```python
from build123d import *

# Parameters (mm, degrees)
BOSS_EXTRUDE1_DEPTH = 6


with BuildPart() as part:
    # Sketch1 → Boss-Extrude1 (new body)
    with BuildSketch(Plane.XY):
        Polygon((349.805861239, 49.832080259), (349.805861239, 56.546676312), (337.582956824, 56.546676312), (337.582956824, 94.832680829), (342.594184557, 99.843908562), (359.928534592, 99.843908562), (364.939762315, 94.832680839), (364.939762315, 73.014449736), (403.254521851, 61.257454897), (403.254521851, 56.546676274), (392.232066466, 56.546676274), (392.232066466, 49.832080221), (403.26125874, 49.832080221), (403.26125874, 24.580912459), (394.140824266, 24.580912459), (337.582956824, 45.121301639), (337.582956824, 49.832080259), align=None)
        Polygon((396.07235895, 38.585081223), (396.445988279, 38.87177709), (396.881088847, 39.052001647), (397.348009271, 39.113472887), (397.814929694, 39.052001647), (398.250030262, 38.87177709), (398.623659591, 38.585081223), (398.910355458, 38.211451895), (399.090580014, 37.776351326), (399.152051254, 37.309430903), (399.090580014, 36.842510479), (398.910355458, 36.407409911), (398.623659591, 36.033780583), (398.250030262, 35.747084715), (397.814929694, 35.566860159), (397.348009271, 35.505388919), (396.881088847, 35.566860159), (396.445988279, 35.747084715), (396.07235895, 36.033780583), (395.785663083, 36.407409911), (395.605438527, 36.842510479), (395.543967287, 37.309430903), (395.605438527, 37.776351326), (395.785663083, 38.211451895), align=None, mode=Mode.SUBTRACT)
        Polygon((351.375405933, 69.514088989), (351.436877173, 69.047168565), (351.617101729, 68.612067997), (351.903797596, 68.238438669), (352.277426924, 67.951742801), (352.712527493, 67.771518245), (353.179447916, 67.710047005), (353.64636834, 67.771518245), (354.081468908, 67.951742801), (354.455098237, 68.238438669), (354.741794104, 68.612067997), (354.92201866, 69.047168565), (354.9834899, 69.514088989), (354.92201866, 69.981009412), (354.741794104, 70.416109981), (354.455098237, 70.789739309), (354.081468908, 71.076435176), (353.64636834, 71.256659733), (353.179447916, 71.318130973), (352.712527493, 71.256659733), (352.277426924, 71.076435176), (351.903797596, 70.789739309), (351.617101729, 70.416109981), (351.436877173, 69.981009412), align=None, mode=Mode.SUBTRACT)
        Polygon((372.381509854, 54.465028594), (372.007880526, 54.751724461), (371.572779958, 54.931949018), (371.105859534, 54.993420258), (370.638939111, 54.931949018), (370.203838542, 54.751724461), (369.830209214, 54.465028594), (369.543513347, 54.091399266), (369.36328879, 53.656298697), (369.30181755, 53.189378274), (369.36328879, 52.72245785), (369.543513347, 52.287357282), (369.830209214, 51.913727954), (370.203838542, 51.627032087), (370.638939111, 51.44680753), (371.105859534, 51.38533629), (371.572779958, 51.44680753), (372.007880526, 51.627032087), (372.381509854, 51.913727954), (372.668205722, 52.287357282), (372.848430278, 52.72245785), (372.909901518, 53.189378274), (372.848430278, 53.656298697), (372.668205722, 54.091399266), align=None, mode=Mode.SUBTRACT)
        Polygon((350.579160049, 82.777243303), (351.409447446, 82.140141376), (352.376337597, 81.739642362), (353.413938539, 81.603039606), (354.45153948, 81.739642362), (355.418429632, 82.140141376), (356.248717028, 82.777243303), (356.885818955, 83.607530699), (357.286317969, 84.574420851), (357.422920725, 85.612021792), (357.286317969, 86.649622733), (356.885818955, 87.616512885), (356.248717028, 88.446800282), (355.418429632, 89.083902209), (354.45153948, 89.484401223), (353.413938539, 89.621003978), (352.376337597, 89.484401223), (351.409447446, 89.083902209), (350.579160049, 88.446800282), (349.942058122, 87.616512885), (349.541559108, 86.649622733), (349.404956353, 85.612021792), (349.541559108, 84.574420851), (349.942058122, 83.607530699), align=None, mode=Mode.SUBTRACT)
    extrude(amount=BOSS_EXTRUDE1_DEPTH)


solid = part.part
```
Geometry check sheet. Reference: the model listing, model coordinates, mm. A direction names the side the tool comes from. Round coordinates to 2 decimals unless told otherwise and drop trailing zeros. Order: outer loops, then holes, each group sorted by start corner. A loop starts at its lowest first (then second) coordinate and runs counter-clockwise, first axis right, second up. Notation, with made-up numbers: (27.5, 46) -> (55.5, 46) arc R16 ccw to (55.5, 67) -> close; hole circle Ø1 at (24.5, 12.25). An arc over 180 degrees is marked (long way). Return JSON: item names as keys, results as strings. Group by question number.
Q1. Section check B-B, the plane z = 4.25. Count the separate pieces of the cut face and the enclosed holes in it, plus the area to 3 significant figures.
Q2. Section check A-A, the plane x = 345.5. Record the boundary of the cut face in (y, z).
Q3. Release check for a two-part mould opening along Y. For faces 4 (the flat face through (344, 56.547, 3)), 5 (the flat face through (364, 63, 0)), 6 (the flat face through (399, 24.581, 3)) record: released by +Y, released by -Y, zero draft, split by the parting line, or undercut.
Q4. Gauge pin test, flat ends, axial feed: pin 1 (3 mm diameter, centred on x = 346.5, z = 2, fed in from -Y); pin 2 (1 mm diameter, centred on x = 375.5, z = 4, fed in from +Y); pin 3 (1.8 mm diameter, centred on y = 88, z = 2.5, fed in from +X); pin 4 (4 mm diameter, centred on x = 365.5, y = 32.5, fed in from +Z). Record the tip position at first contact, or that the pin passes through.
Q5. Material ranges on probe 1 along Y at (x, z) = (398.5, 1.1); probe 2 along X at (y, z) = (77, 4.4); probe 3 along X at (y, z) = (82, 4.75), recorded low to high. Write a range as from..to.
Q6. Section check C-C, the plane x = 377. Record the boundary of the cut face in (y, z), plus the area to 3 significant figures.
Q7. Tool access check on faces 1 (the flat face through (364.94, 84, 3)), 2 (the flat face through (344, 49.832, 3)), 3 (the flat face through (398, 49.832, 3)). Record the directions out of +Z, -Z, +X, -X, +Y, -Y that give a thin tool (end or side, any length) a straight path to the whole face; none if there is none.
Numbers:
{
 "1": {"separate pieces": "1", "enclosed holes": "4", "area": "2,850 mm^2"},
 "2": {"outline": "(42.25, 0) -> (49.83, 0) -> (49.83, 6) -> (42.25, 6) -> close; (56.55, 0) -> (99.84, 0) -> (99.84, 6) -> (56.55, 6) -> close"},
 "3": {"face 4": "undercut", "face 5": "zero draft", "face 6": "released by -Y"},
 "4": {"pin 1": "y = 41.34", "pin 2": "y = 69.93", "pin 3": "x = 364.94", "pin 4": "through"},
 "5": {"probe 1": "24.58..35.94, 38.68..49.83, 56.55..62.72", "probe 2": "337.58..364.94", "probe 3": "337.58..351.75, 355.08..364.94"},
 "6": {"outline": "(30.81, 0) -> (69.31, 0) -> (69.31, 6) -> (30.81, 6) -> close", "area": "231 mm^2"},
 "7": {"face 1": "+Z, -Z, +X, +Y", "face 2": "+Z, -Z, -X", "face 3": "+Z, -Z, +X"}
}
